Autodesk Inventor part; units mm, degrees
ref_plane "YZ Plane" through (0, 0, 0) normal (1, 0, 0) x (0, 1, 0)
ref_plane "XZ Plane" through (0, 0, 0) normal (0, 1, 0) x (-1, 0, 0)
ref_plane "XY Plane" through (0, 0, 0) normal (0, 0, 1) x (1, 0, 0)
sketch "Sketch1" plane through (0, 0, 0) normal (1, 0, 0) x (0, 1, 0)
  circle A0 centre (0, 0) radius 12.95
  line L0 (-1.95, -14) -> (1.95, -14)
  line L1 (1.95, -14) -> (1.95, 14)
  line L2 (1.95, 14) -> (-1.95, 14)
  line L3 (-1.95, 14) -> (-1.95, -14)
  line L4 (-1.95, -14) -> (1.95, 14) construction
  line L5 (1.95, -14) -> (-1.95, 14) construction
  circle A1 centre (0, 0) radius 4.5
  point P0 (1.95, -12.8023)
  point P1 (1.95, 12.8023)
  point P2 (-1.95, 12.8023)
  point P3 (-1.95, -12.8023)
  dimension "d0" = 3.9
  dimension "d1" = 25.9
  dimension "d2" = 28
  dimension "d5" = 9
extrude "Extrusion1" add sketch "Sketch1" along normal blind 1.8 contours A0 L1 A1 | L1 A1 L3 A0 | A0 L3 L2 L1 | L1 L0 L3 A0 | A0 L3 A1 L1 | L3 A1 A0
sketch "Sketch2" plane through (1.8, 0, 0) normal (1, 0, 0) x (0, 0, -1)
  line L0 (7.4, 3.2) -> (7.2, 2.1) construction
  line L1 (6.6621, 3.3342) -> (6.4621, 2.2342)
  line L2 (7.9379, 1.9658) -> (8.1379, 3.0658)
  arc A0 (8.1379, 3.0658) -> (6.6621, 3.3342) centre (7.4, 3.2) ccw
  arc A1 (6.4621, 2.2342) -> (7.9379, 1.9658) centre (7.2, 2.1) ccw
  point P0 (0, 0)
  point P1 (7.3, 2.65)
  dimension "d6" = 0.75
  dimension "d9" = 7.2
  dimension "d10" = 2.1
  dimension "d11" = 7.4
  dimension "d12" = 3.2
extrude "Extrusion2" cut sketch "Sketch2" against normal blind 1.3
sketch "Sketch3" plane through (0, 0, 0) normal (-1, 0, 0) x (0, 0, 1)
  arc A0 (-7.9379, 1.9658) -> (-6.4621, 2.2342) centre (-7.2, 2.1) ccw construction
  line L0 (-8.1379, 3.0658) -> (-7.9379, 1.9658) construction
  arc A1 (-6.6621, 3.3342) -> (-8.1379, 3.0658) centre (-7.4, 3.2) ccw construction
  line L1 (-6.4621, 2.2342) -> (-6.6621, 3.3342) construction
  circle A2 centre (0, 0) radius 9 construction
  line L2 (-7.4, 3.2) -> (-7.2, 2.1) construction
  circle A3 centre (-9.5, 5.5) radius 1
  dimension "d13" = 18
  dimension "d17" = 9.5
  dimension "d18" = 5.5
  dimension "d19" = 2
extrude "Extrusion3" cut sketch "Sketch3" against normal blind 1.3
sketch "Sketch4" plane through (1.3, 5.5, -9.5) normal (-1, 0, 0) x (0, 0, 1)
  circle A0 centre (0, 0) radius 1
  arc A1 (1.5621, -3.5342) -> (3.0379, -3.2658) centre (2.3, -3.4) ccw
  line L0 (1.3621, -2.4342) -> (1.5621, -3.5342)
  arc A2 (2.8379, -2.1658) -> (1.3621, -2.4342) centre (2.1, -2.3) ccw
  line L1 (3.0379, -3.2658) -> (2.8379, -2.1658)
  line L2 (0.7902, 0.6128) -> (2.6927, -1.8404)
  arc A3 (2.8379, -2.1658) -> (1.3621, -2.4342) centre (2.1, -2.3) ccw
  circle A4 centre (0, 0) radius 1
  line L3 (-0.7926, -0.6097) -> (1.7055, -3.8573)
  arc A5 (1.5621, -3.5342) -> (3.0379, -3.2658) centre (2.3, -3.4) ccw
  circle A6 centre (0, 0) radius 1
  point P0 (9.5, -5.5)
  point P1 (2.6927, -1.8404)
  point P2 (-0.7926, -0.6097)
extrude "Extrusion4" cut sketch "Sketch4" along normal up to surface (0.8 mm away) contours A0 L2 A2 L0 A1 L3
pattern_circular "Circular Pattern1" count 2 over 360 about axis through (0, 0, 0) along (1, 0, 0) of "Extrusion2", "Extrusion3", "Extrusion4"
properties part number "ValvePlate"
Design review of the part built by this model. Coordinates are the model's own, in mm. A direction names the side the tool comes from. Round coordinates to 2 decimals unless told otherwise and drop trailing zeros. Write each loop counter-clockwise with the first axis right and the second up, starting at its lowest first coordinate (ties: lowest second). Pieces come first, ordered by that corner, then holes. Notation, with made-up numbers: (8.25, 37.5) - (49.25, 37.5) arc R32 cw to (49.25, 68.5) - close; hole circle Ø8 at (-33, 17.5). An arc over 180 degrees is marked (long way). Use a Markdown table: item, result. Add a question column.
1. Mouldability with a two-part tool opening along Z and no side actions: class faces 1 (the face through (1, 0, -14)), 2 (the face through (1.159, -1.365, 7.05)), 3 (the face through (0.89, -0.59, -4.46)), 4 (the face through (1, -1.95, 13)) as +Z half, -Z half, draft (parallel to the pull), parting line (faces both ways), or undercut.
2. We need section A-A (z = 0). State the section outline as (x, y) points, then the cut area to 3 significant figures.
3. Clearance check with flat-ended pins moving along their axes: pin 1 (1.2 mm diameter, centred on y = -5.5, z = 9.5, fed in from -X); pin 2 (0.6 mm diameter, centred on x = 1, z = -13.5, fed in from +Y). State where each tip first meets the part, or that it passes through.
4. We need section D-D (y = -9.75). State the section outline as (x, z) points.
5. We need section C-C (y = 5.5). State the section outline as (x, z) points.
6. For faces 5 (the face through (1.45, -3.94, 7.29)), 6 (the face through (0.91, -3.29, 9.06)), 7 (the face through (0.496, 6.176, -10.237)), list the 3-axis set-ups (+Z, -Z, +X, -X, +Y, -Y) from which the entire face can be reached by the end or side of a thin tool; tool diameter is ignored.
7. Wall thickness on probe 1 along Z at (x, y) = (1.3, 0); probe 2 along Z at (x, y) = (1.65, 2.5); probe 3 along Y at (x, z) = (0.4, 0): over which ranges is each line inside the solid? List them lowest first.
8. We need section B-B (z = -7.4). State the section outline as (x, y) points, then the cut area to 3 significant figures.
Output:
| question | item | result |
|---|---|---|
| 1 | face 1 | -Z half |
| 1 | face 2 | undercut |
| 1 | face 3 | undercut |
| 1 | face 4 | draft |
| 2 | outline | (0, -12.95) - (1.8, -12.95) - (1.8, -4.5) - (0, -4.5) - close; (0, 4.5) - (1.8, 4.5) - (1.8, 12.95) - (0, 12.95) - close |
| 2 | area | 30.4 mm2 |
| 3 | pin 1 | stops at x = 1.3 |
| 3 | pin 2 | stops at y = 1.95 |
| 4 | outline | (0, -8.52) - (1.8, -8.52) - (1.8, 8.52) - (0, 8.52) - close |
| 5 | outline | (0, -11.72) - (1.8, -11.72) - (1.8, 11.72) - (0, 11.72) - (0, -8.5) - (0.5, -8.5) - (0.5, -8.23) - (1.3, -8.23) - (1.3, -10.5) - (0, -10.5) - close |
| 6 | face 5 | +X |
| 6 | face 6 | none |
| 6 | face 7 | -X |
| 7 | probe 1 | z = -14 to -4.5, 4.5 to 14 |
| 7 | probe 2 | z = -12.71 to -8.04, -6.51 to -3.74, 3.74 to 12.71 |
| 7 | probe 3 | y = -12.95 to -4.5, 4.5 to 12.95 |
| 8 | outline | (0, -10.63) - (1.8, -10.63) - (1.8, 1.38) - (0.5, 1.38) - (0.5, 4.42) - (1.3, 4.42) - (1.3, 3.95) - (1.8, 3.95) - (1.8, 10.63) - (0, 10.63) - close |
| 8 | area | 34.5 mm2 |
